Verification items for the finished model (mm, model axes). A direction names the side the tool comes from. Give positions to 0.01 mm unless a question says otherwise; leave off trailing zeros. Loops run counter-clockwise (first coordinate to the right, second up) from the corner with the lowest first, then second, coordinate; pieces in that order, holes last. Notation, with made-up numbers: (50.25, 42) - (92.25, 42) arc R30 ccw to (92.25, 73) - close; hole circle Ø9 at (69, 15.5). An arc over 180 degrees is marked (long way). One line per question, with ' | ' between items. Start each with the question number.
1. Mould release check, pull along Y, two halves, no side actions. Record for faces 4 (the face through (-13.887, -10.648, 7.395)), 5 (the face through (0, -4, 0)), 6 (the face through (7.09, -5.21, 2.46)): +Y half, -Y half, draft (parallel to the pull), parting line (faces both ways), or undercut.
2. Depth check by flat-ended pin: pin 1 Ø2 at (y, z) = (-12.5, 2) entering from +X; pin 2 Ø1.5 at (x, y) = (6, 6) entering from +Z; pin 3 Ø1.8 at (x, y) = (-5.66, 5.66) entering from -Z. Enter the tip coordinate at first touch or a pass-through.
3. Section check C-C, the plane z = 11.5. Enter the section's corners in (x, y).
4. Section check A-A, the plane y = 0. Enter the section's corners in (x, z).
5. Section check D-D, the plane x = 14. Enter the section's corners in (y, z), then the cut area to 3 significant figures.
6. Tool access check on faces 1 (the face through (6, -6, 10)), 2 (the face through (-0.54, -2.44, 7.4)), 3 (the face through (-5.982, 4.193, 2.465)). Record the directions out of +Z, -Z, +X, -X, +Y, -Y that give a thin tool (end or side, any length) a straight path to the whole face; none if there is none.
7. Thickness scan on line 1 along X through (y, z) = (6, 1); line 2 along X through (y, z) = (-0.5, 10.5); line 3 along X through (y, z) = (6, 12.5). Record the ranges inside material, lowest first. Write a range as from..to.
from build123d import *

# Parameters (mm, degrees)
F0_R          = 17.5
F0_R_2        = 1.5
F0_R_3        = 2.5
F1_DEPTH      = 15
F2_START      = 10
F2_DEPTH      = 15
F3_DEPTH      = 5
F3_DEPTH_BACK = 2


with BuildPart() as f1:
    # F0 (on Top) → F1 (new body)
    with BuildSketch(Plane.XY):
        Circle(F0_R)
        with BuildLine():
            ThreePointArc((-7.1057429889, -5.2686256818), (-5.4610649612, -4.1696869574), (-4.1568542495, -5.6568542495))
            ThreePointArc((-4.1568542495, -5.6568542495), (-4.4668242391, -6.569996393), (-5.2686256818, -7.1057429889))
            ThreePointArc((-5.2686256818, -7.1057429889), (-7.7781745931, -7.7781745931), (-7.1057429889, -5.2686256818))
        make_face(mode=Mode.SUBTRACT)
        with Locations((5.6568542495, -5.6568542495)):
            Circle(F0_R_2, mode=Mode.SUBTRACT)
        with Locations((-5.6568542495, 5.6568542495)):
            Circle(F0_R_2, mode=Mode.SUBTRACT)
        Circle(F0_R_3, mode=Mode.SUBTRACT)
        with BuildLine():
            ThreePointArc((7.1057429889, 5.2686256818), (4.5961940777, 4.5961940777), (5.2686256818, 7.1057429889))
            ThreePointArc((5.2686256818, 7.1057429889), (6.9133037096, 8.2046817133), (8.2175144213, 6.7175144213))
            ThreePointArc((8.2175144213, 6.7175144213), (7.9075444317, 5.8043722778), (7.1057429889, 5.2686256818))
        make_face(mode=Mode.SUBTRACT)
        with Locations((-5.6568542495, 5.6568542495)):
            Circle(F0_R_2)
        with BuildLine():
            ThreePointArc((-5.2686256818, -7.1057429889), (-6.7175144213, -6.7175144213), (-7.1057429889, -5.2686256818))
            ThreePointArc((-7.1057429889, -5.2686256818), (-7.7781745931, -7.7781745931), (-5.2686256818, -7.1057429889))
        make_face()
        with BuildLine():
            ThreePointArc((-5.2175144213, -6.7175144213), (-5.8043722778, -5.5274844108), (-7.1057429889, -5.2686256818))
            ThreePointArc((-7.1057429889, -5.2686256818), (-6.7175144213, -6.7175144213), (-5.2686256818, -7.1057429889))
            ThreePointArc((-5.2686256818, -7.1057429889), (-5.2303471292, -6.9133037096), (-5.2175144213, -6.7175144213))
        make_face()
        with BuildLine():
            ThreePointArc((-5.2686256818, -7.1057429889), (-4.4668242391, -6.569996393), (-4.1568542495, -5.6568542495))
            ThreePointArc((-4.1568542495, -5.6568542495), (-5.4610649612, -4.1696869574), (-7.1057429889, -5.2686256818))
            ThreePointArc((-7.1057429889, -5.2686256818), (-5.8043722778, -5.5274844108), (-5.2175144213, -6.7175144213))
            ThreePointArc((-5.2175144213, -6.7175144213), (-5.2303471292, -6.9133037096), (-5.2686256818, -7.1057429889))
        make_face()
        with Locations((5.6568542495, -5.6568542495)):
            Circle(F0_R_2)
        with BuildLine():
            ThreePointArc((7.1057429889, 5.2686256818), (5.6568542495, 5.6568542495), (5.2686256818, 7.1057429889))
            ThreePointArc((5.2686256818, 7.1057429889), (4.5961940777, 4.5961940777), (7.1057429889, 5.2686256818))
        make_face()
        with BuildLine():
            ThreePointArc((7.1057429889, 5.2686256818), (7.1440215416, 5.4610649612), (7.1568542495, 5.6568542495))
            ThreePointArc((7.1568542495, 5.6568542495), (6.569996393, 6.8468842599), (5.2686256818, 7.1057429889))
            ThreePointArc((5.2686256818, 7.1057429889), (5.6568542495, 5.6568542495), (7.1057429889, 5.2686256818))
        make_face()
        with BuildLine():
            ThreePointArc((5.2686256818, 7.1057429889), (6.569996393, 6.8468842599), (7.1568542495, 5.6568542495))
            ThreePointArc((7.1568542495, 5.6568542495), (7.1440215416, 5.4610649612), (7.1057429889, 5.2686256818))
            ThreePointArc((7.1057429889, 5.2686256818), (7.9075444317, 5.8043722778), (8.2175144213, 6.7175144213))
            ThreePointArc((8.2175144213, 6.7175144213), (6.9133037096, 8.2046817133), (5.2686256818, 7.1057429889))
        make_face()
    extrude(amount=F1_DEPTH)

    # F0 (on Top) → F2 (cut)
    with BuildSketch(Plane.XY.offset(F2_START)):
        with Locations((-5.6568542495, 5.6568542495)):
            Circle(F0_R_2)
        with BuildLine():
            ThreePointArc((7.1057429889, 5.2686256818), (5.6568542495, 5.6568542495), (5.2686256818, 7.1057429889))
            ThreePointArc((5.2686256818, 7.1057429889), (4.5961940777, 4.5961940777), (7.1057429889, 5.2686256818))
        make_face()
        with BuildLine():
            ThreePointArc((7.1057429889, 5.2686256818), (7.1440215416, 5.4610649612), (7.1568542495, 5.6568542495))
            ThreePointArc((7.1568542495, 5.6568542495), (6.569996393, 6.8468842599), (5.2686256818, 7.1057429889))
            ThreePointArc((5.2686256818, 7.1057429889), (5.6568542495, 5.6568542495), (7.1057429889, 5.2686256818))
        make_face()
        with Locations((5.6568542495, -5.6568542495)):
            Circle(F0_R_2)
        with BuildLine():
            ThreePointArc((-5.2686256818, -7.1057429889), (-4.4668242391, -6.569996393), (-4.1568542495, -5.6568542495))
            ThreePointArc((-4.1568542495, -5.6568542495), (-5.4610649612, -4.1696869574), (-7.1057429889, -5.2686256818))
            ThreePointArc((-7.1057429889, -5.2686256818), (-5.8043722778, -5.5274844108), (-5.2175144213, -6.7175144213))
            ThreePointArc((-5.2175144213, -6.7175144213), (-5.2303471292, -6.9133037096), (-5.2686256818, -7.1057429889))
        make_face()
        with BuildLine():
            ThreePointArc((-5.2175144213, -6.7175144213), (-5.8043722778, -5.5274844108), (-7.1057429889, -5.2686256818))
            ThreePointArc((-7.1057429889, -5.2686256818), (-6.7175144213, -6.7175144213), (-5.2686256818, -7.1057429889))
            ThreePointArc((-5.2686256818, -7.1057429889), (-5.2303471292, -6.9133037096), (-5.2175144213, -6.7175144213))
        make_face()
    extrude(amount=F2_DEPTH, mode=Mode.SUBTRACT)

    # F0 (on Top) → F3 (cut, two sides)
    with BuildSketch(Plane.XY) as f3_sk:
        with Locations((-5.6568542495, 5.6568542495)):
            Circle(F0_R_2)
        with Locations((5.6568542495, -5.6568542495)):
            Circle(F0_R_2)
        with BuildLine():
            ThreePointArc((-5.2686256818, -7.1057429889), (-6.7175144213, -6.7175144213), (-7.1057429889, -5.2686256818))
            ThreePointArc((-7.1057429889, -5.2686256818), (-7.7781745931, -7.7781745931), (-5.2686256818, -7.1057429889))
        make_face()
        with BuildLine():
            ThreePointArc((-5.2175144213, -6.7175144213), (-5.8043722778, -5.5274844108), (-7.1057429889, -5.2686256818))
            ThreePointArc((-7.1057429889, -5.2686256818), (-6.7175144213, -6.7175144213), (-5.2686256818, -7.1057429889))
            ThreePointArc((-5.2686256818, -7.1057429889), (-5.2303471292, -6.9133037096), (-5.2175144213, -6.7175144213))
        make_face()
        with BuildLine():
            ThreePointArc((5.2686256818, 7.1057429889), (6.569996393, 6.8468842599), (7.1568542495, 5.6568542495))
            ThreePointArc((7.1568542495, 5.6568542495), (7.1440215416, 5.4610649612), (7.1057429889, 5.2686256818))
            ThreePointArc((7.1057429889, 5.2686256818), (7.9075444317, 5.8043722778), (8.2175144213, 6.7175144213))
            ThreePointArc((8.2175144213, 6.7175144213), (6.9133037096, 8.2046817133), (5.2686256818, 7.1057429889))
        make_face()
        with BuildLine():
            ThreePointArc((7.1057429889, 5.2686256818), (7.1440215416, 5.4610649612), (7.1568542495, 5.6568542495))
            ThreePointArc((7.1568542495, 5.6568542495), (6.569996393, 6.8468842599), (5.2686256818, 7.1057429889))
            ThreePointArc((5.2686256818, 7.1057429889), (5.6568542495, 5.6568542495), (7.1057429889, 5.2686256818))
        make_face()
    extrude(amount=F3_DEPTH, mode=Mode.SUBTRACT)
    extrude(f3_sk.sketch, amount=-F3_DEPTH_BACK, mode=Mode.SUBTRACT)


solid = f1.part
Results list:
1) face 4: parting line | face 5: draft | face 6: undercut
2) pin 1: x = 13.19 | pin 2: z = 10 | pin 3: z = 5
3) outline: circle Ø35 at (0, 0); hole circle Ø3 at (-5.66, -5.66); hole circle Ø3 at (-5.66, 5.66); hole circle Ø5 at (0, 0); hole circle Ø3 at (5.66, -5.66); hole circle Ø3 at (5.66, 5.66)
4) outline: (-17.5, 0) - (-2.5, 0) - (-2.5, 15) - (-17.5, 15) - close; (2.5, 0) - (17.5, 0) - (17.5, 15) - (2.5, 15) - close
5) outline: (-10.5, 0) - (10.5, 0) - (10.5, 15) - (-10.5, 15) - close | area: 315 mm²
6) face 1: +Z | face 2: +Z, -Z | face 3: -Z
7) line 1: -16.44..-7.12, -4.2..5.4, 8.03..16.44 | line 2: -17.49..-2.45, 2.45..17.49 | line 3: -16.44..-7.12, -4.2..4.2, 7.12..16.44
